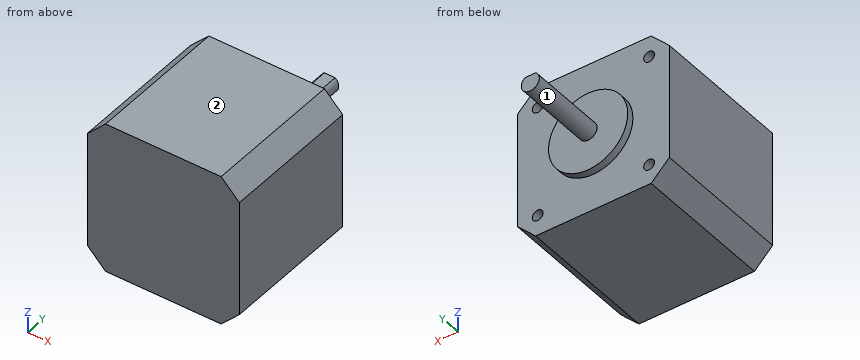
```python
from build123d import *

# Parameters (mm, degrees)
F0_W     = 42.3
F0_H     = 42.3
F1_DEPTH = 39.3
F2_SIZE  = 5.08
F3_R     = 1.5
F4_DEPTH = 3
F5_R     = 11
F6_DEPTH = 2
F8_DEPTH = 22


with BuildPart() as f1:
    # F0 (on Front) → F1 (new body)
    with BuildSketch(Plane.XZ):
        Rectangle(F0_W, F0_H)
    extrude(amount=F1_DEPTH)

    # F2
    f2_edges = [f1.edges().sort_by_distance(p)[0] for p in [
        (-21.15, -19.65, 21.15),
        (21.15, -19.65, 21.15),
        (21.15, -19.65, -21.15),
        (-21.15, -19.65, -21.15),
    ]]
    chamfer(f2_edges, length=F2_SIZE)

    # F3 (on face) → F4 (cut)
    with BuildSketch(Plane(origin=(0, 0, 0), x_dir=(-1, 0, 0), z_dir=(0, 1, 0))):
        with Locations((-15.5, 15.5)):
            Circle(F3_R)
        with Locations((15.5, 15.5)):
            Circle(F3_R)
        with Locations((15.5, -15.5)):
            Circle(F3_R)
        with Locations((-15.5, -15.5)):
            Circle(F3_R)
    extrude(amount=-F4_DEPTH, mode=Mode.SUBTRACT)

    # F5 (on face) → F6 (join)
    with BuildSketch(Plane(origin=(0, 0, 0), x_dir=(-1, 0, 0), z_dir=(0, 1, 0))):
        Circle(F5_R)
    extrude(amount=F6_DEPTH)

    # F7 (on face) → F8 (join)
    with BuildSketch(Plane(origin=(0, 2, 0), x_dir=(-1, 0, 0), z_dir=(0, 1, 0))):
        with BuildLine():
            Line((1.5, 2), (-1.5, 2))
            ThreePointArc((-1.5, 2), (0, -2.5), (1.5, 2))
        make_face()
    extrude(amount=F8_DEPTH)


solid = f1.part
```
Here's how the part is built. I have some questions about the finished solid (model axes, mm). Face numbers are marked on the shaded views. A direction names the side the tool comes from. Coordinates: 2 decimals unless noted, no trailing zeros. Write each loop counter-clockwise with the first axis right and the second up, starting at its lowest first coordinate (ties: lowest second). Pieces come first, ordered by that corner, then holes. Notation, with made-up numbers: (-31.5, 88.5) - (-23.5, 88.5) arc R14 cw to (-23.5, 101.5) - close; hole circle Ø2 at (24, -36). An arc over 180 degrees is marked (long way). One line per item, written item: value.
1) On a 3-axis mill with a long thin cutter (end or side, diameter ignored), from which of +Z, -Z, +X, -X, +Y, -Y can I reach the whole of each face in a straight line? I mean the marked faces 1 and 2. Say none if no direction works.
Model answer:
face 1: +Y
face 2: +Z, +X, -X, +Y, -Y
2) Suppose I cut it at A-A on x = 0. Write out the boundary of the cut face in (y, z), and give its area (3 significant figures).
Model answer:
outline: (-39.3, -21.15) - (0, -21.15) - (0, -11) - (2, -11) - (2, -2.5) - (24, -2.5) - (24, 2) - (2, 2) - (2, 11) - (0, 11) - (0, 21.15) - (-39.3, 21.15) - close
area: 1,810 mm²
3) I'm going to push flat-ended pins straight in: P1, Ø6, axis at x = 15, z = 12.5, coming from the +Y side; P2, Ø0.9, axis at x = 15.5, z = 15.5, coming from the +Y side; P3, Ø17.5, axis at x = 4.5, z = 2.5, coming from the +Y side; P4, Ø10, axis at y = 10, z = 1, coming from the +X side. Where does each tip first touch, or does it pass through?
Model answer:
P1: stops at y = 0
P2: stops at y = -3
P3: stops at y = 24
P4: stops at x = 2.5
4) Suppose I cut it at C-C on y = -19. Write out the boundary of the cut face in (x, z), and give its area (3 significant figures).
Model answer:
outline: (-21.15, -16.07) - (-16.07, -21.15) - (16.07, -21.15) - (21.15, -16.07) - (21.15, 16.07) - (16.07, 21.15) - (-16.07, 21.15) - (-21.15, 16.07) - close
area: 1,740 mm²
5) Suppose I cut it at D-D on y = 1. Write out the boundary of the cut face in (x, z), and give its area (3 significant figures).
Model answer:
outline: circle Ø22 at (0, 0)
area: 380 mm²
6) I need wall thicknesses on line 1 along Z through (x, y) = (-15.5, -1.15); line 2 along Y through (x, z) = (-18, 9.5); line 3 along Y through (x, z) = (1.5, 4). Which ranges of each line are inside material? Lowest first, please.
Model answer:
line 1: z = -21.15 to -17, -14 to 14, 17 to 21.15
line 2: y = -39.3 to 0
line 3: y = -39.3 to 2
7) Suppose I cut it at B-B on z = 0. Write out the boundary of the cut face in (x, y).
Model answer:
outline: (-21.15, -39.3) - (21.15, -39.3) - (21.15, 0) - (11, 0) - (11, 2) - (2.5, 2) - (2.5, 24) - (-2.5, 24) - (-2.5, 2) - (-11, 2) - (-11, 0) - (-21.15, 0) - close
